```python
from build123d import *

# Parameters (mm, degrees)
F0_W     = 152.4
F0_H     = 50.8
F1_DEPTH = 6.35
F3_D     = 6.35
F4_W     = 101.6
F4_H     = 50.8
F5_DEPTH = 127
F7_D     = 31.75
F7_DEPTH = 25.4
F7_TIP   = 9.5386623271
F9_D     = 31.75
F9_DEPTH = 25.4
F9_TIP   = 9.5386623271


with BuildPart() as f1:
    # F0 (on Front) → F1 (new body)
    with BuildSketch(Plane.XZ):
        with Locations((76.2, 25.4)):
            Rectangle(F0_W, F0_H)
    extrude(amount=F1_DEPTH)

    # F3 (through all)
    with Locations(Plane.XZ.offset(6.35)):
        with Locations((12.7, 38.1), (12.7, 12.7), (139.7, 38.1), (139.7, 12.7)):
            Hole(F3_D / 2)

    # F4 (on face) → F5 (join)
    with BuildSketch(Plane.XZ.offset(6.35)):
        with Locations((76.2, 25.4)):
            Rectangle(F4_W, F4_H)
    extrude(amount=F5_DEPTH)

    # F7
    with Locations(Plane.YZ.offset(127)):
        with Locations((-107.95, 25.4)):
            Hole(F7_D / 2, depth=F7_DEPTH)
            with Locations((0, 0, -(F7_DEPTH + F7_TIP / 2))):  # 118° drill point
                Cone(0, F7_D / 2, F7_TIP, mode=Mode.SUBTRACT)

    # F9
    with Locations(Plane(origin=(25.4, 0, 0), x_dir=(0, -1, 0), z_dir=(-1, 0, 0))):
        with Locations((107.95, 25.4)):
            Hole(F9_D / 2, depth=F9_DEPTH)
            with Locations((0, 0, -(F9_DEPTH + F9_TIP / 2))):  # 118° drill point
                Cone(0, F9_D / 2, F9_TIP, mode=Mode.SUBTRACT)


solid = f1.part
```
Input: part model. Units: mm. Frame: model coordinates. A direction names the side the tool comes from. Coordinates: 2 decimals unless noted, no trailing zeros. Write each loop counter-clockwise with the first axis right and the second up, starting at its lowest first coordinate (ties: lowest second). Pieces come first, ordered by that corner, then holes. Notation, with made-up numbers: (-37, -29.5) -> (-8, -29.5) arc R22 cw to (-8, -9.5) -> close; hole circle Ø2 at (84.25, 12.25). An arc over 180 degrees is marked (long way). Answer as a JSON object with one key per item and string values.
1. Mould query, pull axis X, two halves, no side actions, for faces 5 (the face through (10.993, -3.131, 40.777)), 6 (the face through (75, -133.35, 26)), 7 (the face through (25.4, -69, 25)). Classes: released by +X, released by -X, zero draft, split by the parting line, or undercut.
Result set:
{"face 5": "undercut", "face 6": "zero draft", "face 7": "released by -X"}
2. Material intervals for line 1 (Z direction, x = 139.7, y = -1.5) (3 decimals); line 2 (X direction, y = -4, z = 38); line 3 (Z direction, x = 12, y = -2), sorted ascending. Write a range as from..to.
Result set:
{"line 1": "z = 0..9.525, 15.875..34.925, 41.275..50.8", "line 2": "x = 0..9.53, 15.87..136.53, 142.87..152.4", "line 3": "z = 0..9.6, 15.8..35, 41.2..50.8"}
3. Section C-C on x = 98. Return the cut outline in (y, z), then the cut area to 3 significant figures.
Result set:
{"outline": "(-133.35, 0) -> (0, 0) -> (0, 50.8) -> (-133.35, 50.8) -> close; hole circle Ø19.77 at (-107.95, 25.4)", "area": "6,470 mm2"}
4. Section B-B on z = 7.5. Return the cut outline in (x, y).
Result set:
{"outline": "(0, -6.35) -> (25.4, -6.35) -> (25.4, -133.35) -> (127, -133.35) -> (127, -6.35) -> (152.4, -6.35) -> (152.4, 0) -> (0, 0) -> close"}
5. First-contact query: P1, Ø1.5, axis at y = -60.5, z = 44.5, coming from the +X side; P2, Ø7.5, axis at x = 16.5, z = 30.5, coming from the -Y side; P3, Ø5, axis at y = -112.5, z = 34.5, coming from the +X side. Flat tips, straight axial feed; report the tip coordinate or a pass-through.
Result set:
{"P1": "stops at x = 127", "P2": "stops at y = -6.35", "P3": "stops at x = 99.68"}
6. Section D-D on y = -85.5. Return the cut outline in (x, z).
Result set:
{"outline": "(25.4, 0) -> (127, 0) -> (127, 50.8) -> (25.4, 50.8) -> close"}
7. Section A-A on x = 139.7. Return the cut outline in (y, z) (3 decimals), then the cut area to 3 significant figures.
Result set:
{"outline": "(-6.35, 0) -> (0, 0) -> (0, 9.525) -> (-6.35, 9.525) -> close; (-6.35, 15.875) -> (0, 15.875) -> (0, 34.925) -> (-6.35, 34.925) -> close; (-6.35, 41.275) -> (0, 41.275) -> (0, 50.8) -> (-6.35, 50.8) -> close", "area": "242 mm2"}
8. Access query for faces 1 (the face through (13, -6.35, 26)), 2 (the face through (38.28, -92.81, 30.17)), 3 (the face through (140, -6.35, 26)), 4 (the face through (114.12, -92.09, 26.1)). Directions: +Z, -Z, +X, -X, +Y, -Y. A direction counts if a zero-diameter tool reaches every point of the face in a straight line with its end or side. Return the directions, or none.
Result set:
{"face 1": "+Z, -Z, -X, -Y", "face 2": "-X", "face 3": "+Z, -Z, +X, -Y", "face 4": "+X"}
